Can you work these out from the model? Positions are in its coordinate system, mm. A direction names the side the tool comes from. Give positions to 0.01 mm unless a question says otherwise; leave off trailing zeros. Order: outer loops, then holes, each group sorted by start corner. A loop starts at its lowest first (then second) coordinate and runs counter-clockwise, first axis right, second up.
Item 1: I want a section at A-A, the plane x = 0. Write out the boundary of the cut face in (y, z).
Item 2: If we mould it in two halves opening along Z, with no side actions, what happens to faces 4 (the flat face through (2.8, -12, 32)), 5 (the flat face through (0, -11, 14)), 6 (the cylindrical face through (-2.211, -16.021, 33.732)), 7 (the flat face through (-0.1, -10.7, 35))? For each: +Z half, -Z half, draft (parallel to the pull), parting line (faces both ways), or undercut.
Item 3: Which directions (+Z, -Z, +X, -X, +Y, -Y) give clear straight access to the entire face, cutting with the end or side of a thin tool? Please do faces 1 (the flat face through (-5.4, -7, 17)), 2 (the flat face through (4, -8.1, 17)), 3 (the flat face through (-3.7, -9.26, 17.26)).
Item 4: If I drill on line 1 along Z through (x, y) = (0, -6.5); line 2 along Y through (x, z) = (8, 29); line 3 along Y through (x, z) = (0, 10.5), over which ranges is the centre line in solid material (lowest first)?
Item 5: I want a section at D-D, the plane z = 23. Write out the boundary of the cut face in (x, y).
Item 6: I want a section at B-B, the plane z = 8.5. Write out the boundary of the cut face in (x, y).
Item 7: I want a section at C-C, the plane x = 6.5. Write out the boundary of the cut face in (y, z), then the cut area to 3 significant figures.
Item 8: I'm going to push flat-ended pins straight in: pin 1 Ø1.6 at (y, z) = (-7, 11.5) entering from +X; pin 2 Ø3 at (y, z) = (-6, 10) entering from -X; pin 3 Ø2.5 at (x, z) = (-4.5, 13.5) entering from -Y; pin 4 Ø3 at (x, z) = (0, 31.7) entering from +Y. Where does each tip first touch, or does it pass through?
Autodesk Fusion 360 part; units mm, degrees
sketch "Sketch1" plane through (0, 0, 0) normal (0, 0, 1) x (1, 0, 0)
  line L0 (10, 4.8314) -> (10, 9.5)
  line L1 (-4.4022, -9.8222) -> (-3.1214, -8.5414)
  arc A0 (3.2628, -8.2) -> (3.1214, -8.5414) centre (3.2628, -8.4) ccw
  line L2 (-5.5, 6.5607) -> (-5.5, 8.2)
  line L3 (-5.5, -6.5607) -> (-2.8393, -3.9)
  line L4 (-4.8314, 10) -> (-9.5, 10)
  line L5 (2.8393, 3.9) -> (-2.8393, 3.9)
  arc A1 (-10, -9.5) -> (-9.5, -10) centre (-9.5, -9.5) ccw
  line L6 (9.5, 10) -> (4.8314, 10)
  arc A2 (-3.2628, 8.2) -> (-3.1214, 8.5414) centre (-3.2628, 8.4) ccw
  line L7 (-8.2, 3.2628) -> (-8.2, 5.5)
  line L8 (2.8393, -3.9) -> (5.5, -6.5607)
  line L9 (-10, 9.5) -> (-10, 4.9)
  arc A3 (9.5, -10) -> (10, -9.5) centre (9.5, -9.5) ccw
  line L10 (-6.5607, -5.5) -> (-8.2, -5.5)
  line L11 (3.1214, -8.5414) -> (4.2336, -9.6536)
  line L12 (-8.2, -5.5) -> (-8.2, -3.2628)
  line L13 (-9.9987, -4.7917) -> (-10, -9.5)
  line L14 (10, -9.5) -> (10, -4.8314)
  line L15 (3.2628, 8.2) -> (5.5, 8.2)
  arc A4 (8.5414, -3.1214) -> (8.2, -3.2628) centre (8.4, -3.2628) ccw
  arc A5 (-3.1214, -8.5414) -> (-3.2628, -8.2) centre (-3.2628, -8.4) ccw
  line L16 (4.8314, -10) -> (9.5, -10)
  line L17 (-3.9, -2.8393) -> (-6.5607, -5.5)
  line L18 (-3.2628, -8.2) -> (-5.5, -8.2)
  line L19 (3.9, 2.8393) -> (6.5607, 5.5)
  line L20 (-3.1214, 8.5414) -> (-4.4312, 9.8494)
  line L21 (8.2, -5.5) -> (6.5607, -5.5)
  arc A6 (-10, 4.9) -> (-9.8494, 4.4312) centre (-9.3734, 4.8428) ccw
  line L22 (8.5414, 3.1214) -> (9.8222, 4.4022)
  circle A7 centre (0, 0) radius 2.1
  line L23 (3.9, -2.8393) -> (3.9, 2.8393)
  line L24 (6.5607, -5.5) -> (3.9, -2.8393)
  line L25 (5.5, -6.5607) -> (5.5, -8.2)
  line L26 (8.2, -3.2628) -> (8.2, -5.5)
  arc A8 (10, -4.8314) -> (9.8222, -4.4022) centre (9.3929, -4.8314) ccw
  line L27 (-5.5, -8.2) -> (-5.5, -6.5607)
  arc A9 (-4.8314, -10) -> (-4.4022, -9.8222) centre (-4.8314, -9.3929) ccw
  line L28 (5.5, -8.2) -> (3.2628, -8.2)
  line L29 (9.8222, -4.4022) -> (8.5414, -3.1214)
  arc A10 (-9.8222, -4.4022) -> (-9.9987, -4.7917) centre (-9.3929, -4.8314) ccw
  line L30 (-8.5414, -3.1214) -> (-9.8222, -4.4022)
  arc A11 (4.2336, -9.6536) -> (4.8314, -10) centre (4.8837, -9.2207) ccw
  arc A12 (-8.2, -3.2628) -> (-8.5414, -3.1214) centre (-8.4, -3.2628) ccw
  line L31 (-9.5, -10) -> (-4.8314, -10)
  line L32 (-2.8393, -3.9) -> (2.8393, -3.9)
  line L33 (-5.8557, 10) -> (6.4454, 10) construction
  arc A13 (10, 9.5) -> (9.5, 10) centre (9.5, 9.5) ccw
  arc A14 (3.1214, 8.5414) -> (3.2628, 8.2) centre (3.2628, 8.4) ccw
  line L34 (-5.5, 8.2) -> (-3.2628, 8.2)
  line L35 (-3.9, 2.8393) -> (-3.9, -2.8393)
  line L36 (4.4022, 9.8222) -> (3.1214, 8.5414)
  arc A15 (4.8314, 10) -> (4.4022, 9.8222) centre (4.8314, 9.3929) ccw
  line L37 (-9.8494, 4.4312) -> (-8.5414, 3.1214)
  line L38 (5.5, 8.2) -> (5.5, 6.5607)
  line L39 (6.5607, 5.5) -> (8.2, 5.5)
  arc A16 (-8.5414, 3.1214) -> (-8.2, 3.2628) centre (-8.4, 3.2628) ccw
  line L40 (8.2, 5.5) -> (8.2, 3.2628)
  arc A17 (-4.4312, 9.8494) -> (-4.8314, 10) centre (-4.8314, 9.3929) ccw
  line L41 (-8.2, 5.5) -> (-6.5607, 5.5)
  arc A18 (9.8222, 4.4022) -> (10, 4.8314) centre (9.3929, 4.8314) ccw
  arc A19 (-9.5, 10) -> (-10, 9.5) centre (-9.5, 9.5) ccw
  line L42 (-2.8393, 3.9) -> (-5.5, 6.5607)
  line L43 (-6.5607, 5.5) -> (-3.9, 2.8393)
  arc A20 (8.2, 3.2628) -> (8.5414, 3.1214) centre (8.4, 3.2628) ccw
  line L44 (5.5, 6.5607) -> (2.8393, 3.9)
  line L45 (5.4, -6.6021) -> (5.4, -8.1)
  line L46 (5.4, -8.1) -> (3.2628, -8.1)
  arc A21 (3.2628, -8.1) -> (3.0507, -8.6121) centre (3.2628, -8.4) ccw
  line L47 (3.0507, -8.6121) -> (4.1561, -9.7175)
  arc A22 (4.1561, -9.7175) -> (4.8282, -10.1) centre (4.8837, -9.2207) ccw
  line L48 (4.8282, -10.1) -> (9.5, -10.1)
  arc A23 (9.5, -10.1) -> (10.1, -9.5) centre (9.5, -9.5) ccw
  line L49 (10.1, -9.5) -> (10.1, -4.8314)
  arc A24 (10.1, -4.8314) -> (9.8929, -4.3315) centre (9.3929, -4.8314) ccw
  line L50 (9.8929, -4.3315) -> (8.6121, -3.0507)
  arc A25 (8.6121, -3.0507) -> (8.1, -3.2628) centre (8.4, -3.2628) ccw
  line L51 (8.1, -3.2628) -> (8.1, -5.4)
  line L52 (8.1, -5.4) -> (6.6021, -5.4)
  line L53 (6.6021, -5.4) -> (4, -2.7979)
  line L54 (4, -2.7979) -> (4, 2.7979)
  line L55 (4, 2.7979) -> (6.6021, 5.4)
  line L56 (6.6021, 5.4) -> (8.1, 5.4)
  line L57 (8.1, 5.4) -> (8.1, 3.2628)
  arc A26 (8.1, 3.2628) -> (8.6121, 3.0507) centre (8.4, 3.2628) ccw
  line L58 (8.6121, 3.0507) -> (9.8929, 4.3315)
  arc A27 (9.8929, 4.3315) -> (10.1, 4.8314) centre (9.3929, 4.8314) ccw
  line L59 (10.1, 4.8314) -> (10.1, 9.5)
  arc A28 (10.1, 9.5) -> (9.5, 10.1) centre (9.5, 9.5) ccw
  line L60 (9.5, 10.1) -> (4.8314, 10.1)
  arc A29 (4.8314, 10.1) -> (4.3315, 9.8929) centre (4.8314, 9.3929) ccw
  line L61 (4.3315, 9.8929) -> (3.0507, 8.6121)
  arc A30 (3.0507, 8.6121) -> (3.2628, 8.1) centre (3.2628, 8.4) ccw
  line L62 (3.2628, 8.1) -> (5.4, 8.1)
  line L63 (5.4, 8.1) -> (5.4, 6.6021)
  line L64 (5.4, 6.6021) -> (2.7979, 4)
  line L65 (2.7979, 4) -> (-2.7979, 4)
  line L66 (-2.7979, 4) -> (-5.4, 6.6021)
  line L67 (-5.4, 6.6021) -> (-5.4, 8.1)
  line L68 (-5.4, 8.1) -> (-3.2628, 8.1)
  arc A31 (-3.2628, 8.1) -> (-3.0509, 8.6124) centre (-3.2628, 8.4) ccw
  line L69 (-3.0509, 8.6124) -> (-4.3627, 9.9223)
  arc A32 (-4.3627, 9.9223) -> (-4.8314, 10.1) centre (-4.8314, 9.3929) ccw
  line L70 (-4.8314, 10.1) -> (-9.5, 10.1)
  arc A33 (-9.5, 10.1) -> (-10.1, 9.5) centre (-9.5, 9.5) ccw
  line L71 (-10.1, 9.5) -> (-10.1, 4.9044)
  arc A34 (-10.1, 4.9044) -> (-9.9226, 4.363) centre (-9.3734, 4.8428) ccw
  line L72 (-9.9226, 4.363) -> (-8.6124, 3.0509)
  arc A35 (-8.6124, 3.0509) -> (-8.1, 3.2628) centre (-8.4, 3.2628) ccw
  line L73 (-8.1, 3.2628) -> (-8.1, 5.4)
  line L74 (-8.1, 5.4) -> (-6.6021, 5.4)
  line L75 (-6.6021, 5.4) -> (-4, 2.7979)
  line L76 (-4, 2.7979) -> (-4, -2.7979)
  line L77 (-4, -2.7979) -> (-6.6021, -5.4)
  line L78 (-6.6021, -5.4) -> (-8.1, -5.4)
  line L79 (-8.1, -5.4) -> (-8.1, -3.2628)
  arc A36 (-8.1, -3.2628) -> (-8.6121, -3.0507) centre (-8.4, -3.2628) ccw
  line L80 (-8.6121, -3.0507) -> (-9.8929, -4.3315)
  arc A37 (-9.8929, -4.3315) -> (-10.0987, -4.7886) centre (-9.3929, -4.8314) ccw
  line L81 (-10.0987, -4.7886) -> (-10.1, -9.4997)
  arc A38 (-10.1, -9.4997) -> (-9.5, -10.1) centre (-9.5, -9.5) ccw
  line L82 (-9.5, -10.1) -> (-4.8314, -10.1)
  arc A39 (-4.8314, -10.1) -> (-4.3315, -9.8929) centre (-4.8314, -9.3929) ccw
  line L83 (-4.3315, -9.8929) -> (-3.0507, -8.6121)
  arc A40 (-3.0507, -8.6121) -> (-3.2628, -8.1) centre (-3.2628, -8.4) ccw
  line L84 (-3.2628, -8.1) -> (-5.4, -8.1)
  line L85 (-5.4, -8.1) -> (-5.4, -6.6021)
  line L86 (-5.4, -6.6021) -> (-2.7979, -4)
  line L87 (-2.7979, -4) -> (2.7979, -4)
  line L88 (2.7979, -4) -> (5.4, -6.6021)
  line L89 (-9.5, -9.5) -> (9.5, -9.5)
  line L90 (9.5, -9.5) -> (9.5, -17.5)
  line L91 (9.5, -17.5) -> (-9.5, -17.5)
  line L92 (-9.5, -17.5) -> (-9.5, -9.5)
  dimension "d1" = 0.1
  dimension "d2" = 8
extrude "Extrude1" add sketch "Sketch1" along normal blind 35 contours L47 A22 L48 L82 A39 L83 L89 L90 L91 L92 | L45 L46 A21 L47 L83 A40 L84 L85 L86 L87 L88 L89
sketch "Sketch2" plane through (0, -17.5, 0) normal (0, -1, 0) x (1, 0, 0)
  line L0 (-9.5, 0) -> (9.5, 0)
  line L1 (9.5, 0) -> (9.5, 35)
  line L2 (9.5, 35) -> (-9.5, 35)
  line L3 (-9.5, 35) -> (-9.5, 0)
  line L4 (-9.5114, 14.292) -> (9.5, 17.5) construction
  line L5 (13.7765, 12.4651) -> (0.5613, -1.2651)
  line L6 (0.5613, -1.2651) -> (-13.7765, 12.5349)
  line L7 (-13.7765, 12.5349) -> (-0.5613, 26.2651)
  line L8 (-0.5613, 26.2651) -> (13.7765, 12.4651)
  line L9 (13.7765, 12.4651) -> (-13.7765, 12.5349) construction
  line L10 (0.5613, -1.2651) -> (-0.5613, 26.2651) construction
  line L11 (-0.5613, 26.2651) -> (-5.901, 20.7173) construction
  line L12 (-5.901, 20.7173) -> (8.4368, 6.9173) construction
  line L13 (-5.901, 20.7173) -> (-2.1905, 17.1459) construction
  line L14 (-2.1905, 17.1459) -> (4.7263, 10.4887) construction
  line L15 (4.7263, 10.4887) -> (8.4368, 6.9173) construction
  circle A0 centre (-2.1905, 17.1459) radius 1.05
  circle A1 centre (4.7263, 10.4887) radius 1.05
  line L16 (-0.5613, 26.2651) -> (8.1636, 35.3299)
  point P0 (0, 12.5)
  dimension "d5" = 19.9
  dimension "d6" = 7.7
  dimension "d7" = 5.15
  dimension "d8" = 9.6
  dimension "d9" = 5.15
  dimension "d10" = 2.1
  dimension "d11" = 2.1
extrude "Extrude2" cut sketch "Sketch2" against normal blind 6.5 contours L0 L3 L6 | L0 L1 L3 L5 L6 L7 L8 | L1 L2 L8 L16
sketch "Sketch3" plane through (0, -17.5, 0) normal (0, -1, 0) x (1, 0, 0)
  line L0 (-9.5, 16.978) -> (7.846, 35)
  line L1 (7.846, 35) -> (-9.5, 35)
  line L2 (-9.5, 35) -> (-9.5, 16.978)
  circle A0 centre (0, 31.7046) radius 1.55
  circle A1 centre (0, 31.7046) radius 3
  line L3 (-9.5, 35) -> (0, 35) construction
  line L4 (0, 35) -> (0, 26.8482) construction
  line L5 (0, 30.9241) -> (-9.5, 30.9241) construction
  dimension "d14" = 3.1
  dimension "d15" = 6
  dimension "d16" = 9.5
extrude "Extrude3" cut sketch "Sketch3" against normal blind 20 contours A0
extrude "Extrude4" cut sketch "Sketch3" against normal blind 3 contours A1
sketch "Sketch4" plane through (0, 0, 35) normal (0, 0, 1) x (-1, 0, 0)
  line L0 (-7.846, 17.5) -> (-7.846, 11)
  line L1 (-7.846, 11) -> (-9.5, 11)
  line L2 (-9.5, 11) -> (-9.5, 10.1)
  line L3 (-9.5, 10.1) -> (-4.8282, 10.1)
  arc A0 (-4.1561, 9.7175) -> (-4.8282, 10.1) centre (-4.8837, 9.2207) ccw
  line L4 (-4.1561, 9.7175) -> (-3.0507, 8.6121)
  arc A1 (-3.2628, 8.1) -> (-3.0507, 8.6121) centre (-3.2628, 8.4) ccw
  line L5 (-3.2628, 8.1) -> (-5.4, 8.1)
  line L6 (-5.4, 8.1) -> (-5.4, 6.6021)
  line L7 (-5.4, 6.6021) -> (-2.7979, 4)
  line L8 (-2.7979, 4) -> (2.7979, 4)
  line L9 (2.7979, 4) -> (5.4, 6.6021)
  line L10 (5.4, 6.6021) -> (5.4, 8.1)
  line L11 (5.4, 8.1) -> (3.2628, 8.1)
  arc A2 (3.0507, 8.6121) -> (3.2628, 8.1) centre (3.2628, 8.4) ccw
  line L12 (3.0507, 8.6121) -> (4.3315, 9.8929)
  arc A3 (4.8314, 10.1) -> (4.3315, 9.8929) centre (4.8314, 9.3929) ccw
  line L13 (4.8314, 10.1) -> (9.5, 10.1)
  line L14 (9.5, 10.1) -> (9.5, 17.5)
  line L15 (9.5, 17.5) -> (-7.846, 17.5)
  line L16 (2.8, 11.05) -> (-2.8, 11.05)
  line L17 (-2.8, 11.05) -> (-2.8, 12.95)
  line L18 (-2.8, 12.95) -> (2.8, 12.95)
  line L19 (2.8, 12.95) -> (2.8, 11.05)
  line L20 (2.8, 11.05) -> (-2.8, 12.95) construction
  line L21 (-2.8, 11.05) -> (2.8, 12.95) construction
  line L22 (9.5, 10.5577) -> (-9.5, 10.55) construction
  line L23 (0, 12) -> (0, 17.5) construction
  point P0 (0, 12)
  dimension "d21" = 5.6
  dimension "d22" = 1.9
  dimension "d25" = 5.5
extrude "Extrude5" cut sketch "Sketch4" against normal blind 6.5 contours L16 L17 L18 L19
Results list:
1. outline: (-17.5, 26.85) - (-11, 26.85) - (-11, 0) - (-4, 0) - (-4, 30.15) - (-11.05, 30.15) - (-11.05, 28.5) - (-12.95, 28.5) - (-12.95, 30.15) - (-14.5, 30.15) - (-14.5, 28.7) - (-17.5, 28.7) - close; (-17.5, 34.7) - (-14.5, 34.7) - (-14.5, 33.25) - (-12.95, 33.25) - (-12.95, 35) - (-17.5, 35) - close; (-11.05, 33.25) - (-4, 33.25) - (-4, 35) - (-11.05, 35) - close
2. face 4: draft
2. face 5: undercut
2. face 6: undercut
2. face 7: +Z half
3. face 1: +Z, -Z, -X, +Y
3. face 2: +Z, -Z, +X
3. face 3: +Z, -Z, -X
4. line 1: z = 0 to 30.15, 33.25 to 35
4. line 2: y = -11 to -10.1
4. line 3: y = -11 to -4
5. outline: (-9.5, -17.5) - (-3.7, -17.5) - (-3.7, -11) - (9.5, -11) - (9.5, -10.1) - (4.83, -10.1) arc R0.88 cw to (4.16, -9.72) - (3.05, -8.61) arc R0.3 cw to (3.26, -8.1) - (5.4, -8.1) - (5.4, -6.6) - (2.8, -4) - (-2.8, -4) - (-5.4, -6.6) - (-5.4, -8.1) - (-3.26, -8.1) arc R0.3 cw to (-3.05, -8.61) - (-4.33, -9.89) arc R0.71 cw to (-4.83, -10.1) - (-9.5, -10.1) - close
6. outline: (-9.5, -11) - (9.5, -11) - (9.5, -10.1) - (4.83, -10.1) arc R0.88 cw to (4.16, -9.72) - (3.05, -8.61) arc R0.3 cw to (3.26, -8.1) - (5.4, -8.1) - (5.4, -6.6) - (2.8, -4) - (-2.8, -4) - (-5.4, -6.6) - (-5.4, -8.1) - (-3.26, -8.1) arc R0.3 cw to (-3.05, -8.61) - (-4.33, -9.89) arc R0.71 cw to (-4.83, -10.1) - (-9.5, -10.1) - close
7. outline: (-17.5, 0) - (-10.1, 0) - (-10.1, 35) - (-17.5, 35) - (-17.5, 33.6) - (-11, 33.6) - (-11, 4.91) - (-17.5, 4.91) - close
7. area: 72.5 mm2
8. pin 1: stops at x = 5.4
8. pin 2: stops at x = -5.4
8. pin 3: stops at y = -11
8. pin 4: passes through
